```python
from build123d import *

# Parameters (mm, degrees)
SCHIZZO1_W                  = 290
SCHIZZO1_H                  = 200
ESTRUSIONE1_DEPTH           = 20
M10_TAPPED_HOLE1_AT_2_COUNT = 2
M10_TAPPED_HOLE1_AT_2_PITCH = 168
M10_TAPPED_HOLE1_AT_3_COUNT = 2
M10_TAPPED_HOLE1_AT_3_PITCH = 126
M10_TAPPED_HOLE1_AT_4_COUNT = 2
M10_TAPPED_HOLE1_AT_4_PITCH = 42
M10_TAPPED_HOLE1_AT_5_COUNT = 2
M10_TAPPED_HOLE1_AT_5_PITCH = 84
M14_TAPPED_HOLE1_D          = 12
M14_TAPPED_HOLE1_DEPTH      = 38
M14_TAPPED_HOLE1_TIP        = 3.605163714
SMUSSO1_SIZE                = 2


with BuildPart() as part:
    # Schizzo1 → Estrusione1 (new body)
    with BuildSketch(Plane(origin=(0, 0, 0), x_dir=(0, 0, -1), z_dir=(1, 0, 0))):
        with Locations((145, 100)):
            Rectangle(SCHIZZO1_W, SCHIZZO1_H)
    extrude(amount=ESTRUSIONE1_DEPTH)

    # Schizzo2 → M10 Tapped Hole1 (revolve, cut)
    with BuildSketch(Plane(origin=(10, 184, 0), x_dir=(0, -1, 0), z_dir=(1, 0, 0))):
        Polygon((0, 0), (0, 30.053657631), (4.25, 27.5), (4.25, 0), align=None)
    m10_tapped_hole1 = revolve(axis=Axis((10, 184, 6.35), (0, 0, -1)), mode=Mode.SUBTRACT)

    # M10 Tapped Hole1 at 2: M10 Tapped Hole1 ×2
    with Locations(*[(0, -i * M10_TAPPED_HOLE1_AT_2_PITCH, 0) for i in range(1, M10_TAPPED_HOLE1_AT_2_COUNT)]):
        add(m10_tapped_hole1, mode=Mode.SUBTRACT)

    # M10 Tapped Hole1 at 3: M10 Tapped Hole1 ×2
    with Locations(*[(0, -i * M10_TAPPED_HOLE1_AT_3_PITCH, 0) for i in range(1, M10_TAPPED_HOLE1_AT_3_COUNT)]):
        add(m10_tapped_hole1, mode=Mode.SUBTRACT)

    # M10 Tapped Hole1 at 4: M10 Tapped Hole1 ×2
    with Locations(*[(0, -i * M10_TAPPED_HOLE1_AT_4_PITCH, 0) for i in range(1, M10_TAPPED_HOLE1_AT_4_COUNT)]):
        add(m10_tapped_hole1, mode=Mode.SUBTRACT)

    # M10 Tapped Hole1 at 5: M10 Tapped Hole1 ×2
    with Locations(*[(0, -i * M10_TAPPED_HOLE1_AT_5_PITCH, 0) for i in range(1, M10_TAPPED_HOLE1_AT_5_COUNT)]):
        add(m10_tapped_hole1, mode=Mode.SUBTRACT)

    # Specchia1: M10 Tapped Hole1 across plane
    add(m10_tapped_hole1.mirror(Plane.XY.offset(-145)), mode=Mode.SUBTRACT)

    # Specchia1 copy 1 sketch → Specchia1 copy 1 (revolve, cut)
    with BuildSketch(Plane(origin=(10, 16, -290), x_dir=(0, -1, 0), z_dir=(1, 0, 0))):
        Polygon((0, 0), (0, -30.053657631), (4.25, -27.5), (4.25, 0), align=None)
    revolve(axis=Axis((10, 16, -296.35), (0, 0, -1)), mode=Mode.SUBTRACT)

    # Specchia1 copy 2 sketch → Specchia1 copy 2 (revolve, cut)
    with BuildSketch(Plane(origin=(10, 58, -290), x_dir=(0, -1, 0), z_dir=(1, 0, 0))):
        Polygon((0, 0), (0, -30.053657631), (4.25, -27.5), (4.25, 0), align=None)
    revolve(axis=Axis((10, 58, -296.35), (0, 0, -1)), mode=Mode.SUBTRACT)

    # Specchia1 copy 3 sketch → Specchia1 copy 3 (revolve, cut)
    with BuildSketch(Plane(origin=(10, 142, -290), x_dir=(0, -1, 0), z_dir=(1, 0, 0))):
        Polygon((0, 0), (0, -30.053657631), (4.25, -27.5), (4.25, 0), align=None)
    revolve(axis=Axis((10, 142, -296.35), (0, 0, -1)), mode=Mode.SUBTRACT)

    # Specchia1 copy 4 sketch → Specchia1 copy 4 (revolve, cut)
    with BuildSketch(Plane(origin=(10, 100, -290), x_dir=(0, -1, 0), z_dir=(1, 0, 0))):
        Polygon((0, 0), (0, -30.053657631), (4.25, -27.5), (4.25, 0), align=None)
    revolve(axis=Axis((10, 100, -296.35), (0, 0, -1)), mode=Mode.SUBTRACT)

    # M14 Tapped Hole1
    with Locations(Plane(origin=(20, 0, 0), x_dir=(0, 0, -1), z_dir=(1, 0, 0))):
        with Locations((35, 14), (255, 14)):
            Hole(M14_TAPPED_HOLE1_D / 2, depth=M14_TAPPED_HOLE1_DEPTH)
            with Locations((0, 0, -(M14_TAPPED_HOLE1_DEPTH + M14_TAPPED_HOLE1_TIP / 2))):  # 118° drill point
                Cone(0, M14_TAPPED_HOLE1_D / 2, M14_TAPPED_HOLE1_TIP, mode=Mode.SUBTRACT)

    # Smusso1
    smusso1_edges = [part.edges().sort_by_distance(p)[0] for p in [
        (0, 200, -145),
    ]]
    chamfer(smusso1_edges, length=SMUSSO1_SIZE)


solid = part.part
```
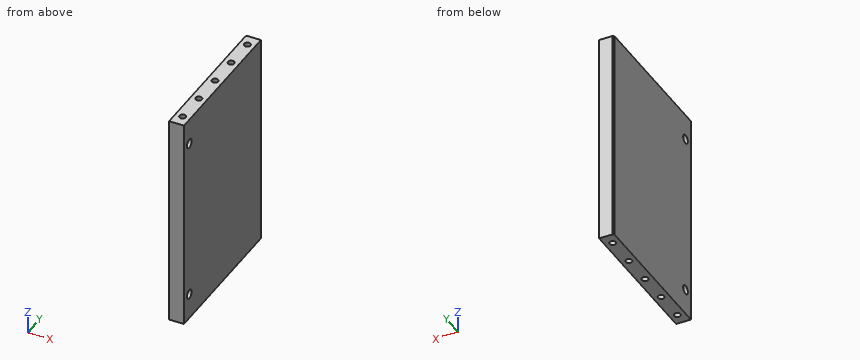
Could you check a few things on this model? Use its own coordinates, in mm. Round coordinates to 2 decimals unless told otherwise and drop trailing zeros. Loops run counter-clockwise (first coordinate to the right, second up) from the corner with the lowest first, then second, coordinate; pieces in that order, holes last. Notation, with made-up numbers: (-9.5, 66.5) - (42.5, 66.5) arc R24 ccw to (42.5, 83.5) - close; hole circle Ø2 at (33.25, 44). An arc over 180 degrees is marked (long way). Use CSV: the item, a comma, the result in double quotes.
Item 1: If we section it at B-B on z = -270: List the corners of the cut face in (x, y) for me.
Here are the results:
outline,"(0, 0) - (20, 0) - (20, 200) - (2, 200) - (0, 198) - close; hole circle Ø8.5 at (10, 16); hole circle Ø8.5 at (10, 58); hole circle Ø8.5 at (10, 100); hole circle Ø8.5 at (10, 142); hole circle Ø8.5 at (10, 184)"
Item 2: Will these pins go through, and if not, where does the flat tip stop? pin 1 (7 mm diameter, centred on x = 10, y = 184, fed in from +Z); pin 2 (5 mm diameter, centred on x = 10, y = 100, fed in from -Z); pin 3 (7 mm diameter, centred on x = 10, y = 58, fed in from -Z).
Here are the results:
pin 1,"stops at z = -27.95"
pin 2,"stops at z = -261.45"
pin 3,"stops at z = -262.05"
Item 3: I need wall thicknesses on L1, parallel to Y at x = 10, z = -278; L2, parallel to Y at x = 10.5, z = -35; L3, parallel to X at y = 58, z = -272. Which ranges of each line are inside material? Lowest first, please. Write a range as [from, to].
Here are the results:
L1,"y = [0, 11.75], [20.25, 53.75], [62.25, 95.75], [104.25, 137.75], [146.25, 179.75], [188.25, 200]"
L2,"y = [0, 8], [20, 200]"
L3,"x = [0, 5.75], [14.25, 20]"
Item 4: If we section it at A-A on z = -35: List the corners of the cut face in (x, y) for me.
Here are the results:
outline,"(0, 0) - (20, 0) - (20, 8) - (0, 8) - close; (0, 20) - (20, 20) - (20, 200) - (2, 200) - (0, 198) - close"
